Build history of the part. All positions in model axes, mm. A direction names the side the tool comes from. Give positions to 0.01 mm unless a question says otherwise; leave off trailing zeros. Write each loop counter-clockwise with the first axis right and the second up, starting at its lowest first coordinate (ties: lowest second). Pieces come first, ordered by that corner, then holes. Notation, with made-up numbers: M 2.5,89.5 L 37.5,89.5 A33 ccw 37.5,118.5 Z; hole C 52,-40 d3. An arc over 180 degrees is marked long. Return JSON: item names as keys, results as strings. Group by question number.
Q1. Band-saw the part on B-B, the plane z = 36. Give the cut face in (x, y).
Q2. Band-saw the part on C-C, the plane x = 7. Give the cut face in (y, z).
Q3. Band-saw the part on A-A, the plane y = 16.5. Give the cut face in (x, z).
Q4. Flat gauge pins, fed straight in: pin 1 Ø1 at (y, z) = (57, 36) entering from -X; pin 2 Ø2 at (y, z) = (125, 11.5) entering from +X; pin 3 Ø10 at (x, y) = (19, 65.5) entering from -Z. Where does each tip first touch, or does it go through?
Q5. Tool access for faces 1 (the flat face through (13, 51, -49.258)), 2 (the flat face through (22.246, -140, 13)), 3 (the flat face through (13, 51, 49.258)), 4 (the flat face through (-22.246, 86, 13)): list every direction of +Z, -Z, +X, -X, +Y, -Y with a clear straight run to the whole face (end or side of a thin tool).
Q6. Band-saw the part on D-D, the plane z = 8.5. Give the cut face in (x, y).
Q7. Wall check: probe 1 along Y at (x, z) = (61, 24.5); probe 2 along X at (y, z) = (-96, -6); probe 3 along Z at (x, y) = (12.5, 53). Give the ranges that are in metal, low to high.
from build123d import *

# Parameters (mm, degrees)
F0_W     = 206.809192
F0_H     = 98.516002
F3_DEPTH = 25.4
F1_W     = 334.808738
F1_H     = 115.25692
F4_DEPTH = 25.4
F2_W     = 44.491924
F2_H     = 350.738764
F5_DEPTH = 25.4


with BuildPart() as f3:
    # F0 (on Right) → F3 (new body)
    with BuildSketch(Plane.YZ):
        Rectangle(F0_W, F0_H)
    extrude(amount=F3_DEPTH)

    # F1 (on Front) → F4 (join)
    with BuildSketch(Plane.XZ):
        Rectangle(F1_W, F1_H)
    extrude(amount=F4_DEPTH)

    # F2 (on Top) → F5 (join)
    with BuildSketch(Plane.XY):
        Rectangle(F2_W, F2_H)
    extrude(amount=F5_DEPTH)


solid = f3.part
From the geometry:
{
 "1": {"outline": "M -167.4,-25.4 L 0,-25.4 L 0,-103.4 L 25.4,-103.4 L 25.4,-25.4 L 167.4,-25.4 L 167.4,0 L 25.4,0 L 25.4,103.4 L 0,103.4 L 0,0 L -167.4,0 Z"},
 "2": {"outline": "M -175.37,0 L -103.4,0 L -103.4,-49.26 L -25.4,-49.26 L -25.4,-57.63 L 0,-57.63 L 0,-49.26 L 103.4,-49.26 L 103.4,0 L 175.37,0 L 175.37,25.4 L 103.4,25.4 L 103.4,49.26 L 0,49.26 L 0,57.63 L -25.4,57.63 L -25.4,49.26 L -103.4,49.26 L -103.4,25.4 L -175.37,25.4 Z"},
 "3": {"outline": "M -22.25,0 L 0,0 L 0,-49.26 L 25.4,-49.26 L 25.4,49.26 L 0,49.26 L 0,25.4 L -22.25,25.4 Z"},
 "4": {"pin 1": "stops at x = 0", "pin 2": "stops at x = 22.25", "pin 3": "stops at z = -49.26"},
 "5": {"face 1": "-Z, +X, -X, +Y", "face 2": "+Z, -Z, +X, -Y", "face 3": "+Z, +X, -X, +Y", "face 4": "+Z, -Z, -X, +Y"},
 "6": {"outline": "M -167.4,-25.4 L -22.25,-25.4 L -22.25,-175.37 L 22.25,-175.37 L 22.25,-103.4 L 25.4,-103.4 L 25.4,-25.4 L 167.4,-25.4 L 167.4,0 L 25.4,0 L 25.4,103.4 L 22.25,103.4 L 22.25,175.37 L -22.25,175.37 L -22.25,0 L -167.4,0 Z"},
 "7": {"probe 1": "y = -25.4 to 0", "probe 2": "x = 0 to 25.4", "probe 3": "z = -49.26 to 49.26"}
}
